Could you check a few things on this model? Use its own coordinates, in mm. Face numbers are marked on the shaded views. A direction names the side the tool comes from. Give positions to 0.01 mm unless a question says otherwise; leave off trailing zeros. Write each loop counter-clockwise with the first axis right and the second up, starting at its lowest first coordinate (ties: lowest second). Pieces come first, ordered by that corner, then holes. Notation, with made-up numbers: (-17, 24) - (22, 24) arc R31 ccw to (22, 62) - close; hole circle Ø4 at (79, 41). An arc over 180 degrees is marked (long way). Write item = value, one per line.
from build123d import *

# Parameters (mm, degrees)
F0_W     = 762
F0_H     = 762
F1_DEPTH = 155.448
F3_DEPTH = 128.016


with BuildPart() as f1:
    # F0 (on Front) → F1 (new body)
    with BuildSketch(Plane.XZ):
        with Locations((-381, 381)):
            Rectangle(F0_W, F0_H)
    extrude(amount=F1_DEPTH)

    # F2 (on face) → F3 (cut)
    with BuildSketch(Plane.XZ.offset(155.448)):
        Polygon((-747.250676, 388.62), (-381, 388.62), (-11.85805, 388.62), (-11.85805, 749.354362), (-747.250676, 749.354362), align=None)
        Polygon((-381, 373.38), (-747.250676, 373.38), (-747.250676, 13.386413), (-11.85805, 13.386413), (-11.85805, 373.38), align=None)
    extrude(amount=-F3_DEPTH, mode=Mode.SUBTRACT)


solid = f1.part
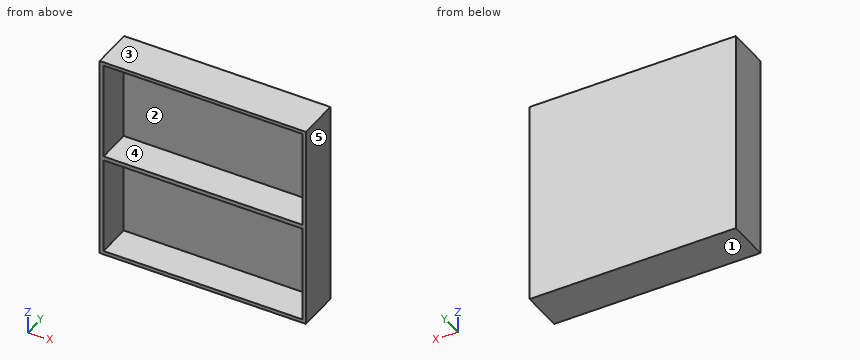
1. Which directions (+Z, -Z, +X, -X, +Y, -Y) give clear straight access to the entire face, cutting with the end or side of a thin tool? Please do the marked faces 1 and 2.
Filled sheet:
face_1 = -Z, +X, -X, +Y, -Y
face_2 = -Y
2. Thinking about a two-plate mould opening in X: for the marked faces 3, 4 and 5, which applies, pulls with the +X half, pulls with the -X half, needs draft (parallel to the pull), parting line crosses it, or undercut?
Filled sheet:
face_3 = needs draft
face_4 = undercut
face_5 = pulls with the +X half
3. For pin 1 (5 mm diameter, centred on x = -117, z = 569.5, fed in from -Y), with a flat end and sliding along its axis, tell me the tip position at first contact or that it passes through.
Filled sheet:
pin_1 = -27.43
4. If we section it at C-C, the plane z = 597.5: Please give me the cut outline in (x, y), and give its area (3 significant figures).
Filled sheet:
outline = (-762, -155.45) - (-747.25, -155.45) - (-747.25, -27.43) - (-11.86, -27.43) - (-11.86, -155.45) - (0, -155.45) - (0, 0) - (-762, 0) - close
area = 24,300 mm2
5. If we section it at B-B, the plane x = -407: Please give me the cut outline in (y, z).
Filled sheet:
outline = (-155.45, 0) - (0, 0) - (0, 762) - (-155.45, 762) - (-155.45, 749.35) - (-27.43, 749.35) - (-27.43, 388.62) - (-155.45, 388.62) - (-155.45, 373.38) - (-27.43, 373.38) - (-27.43, 13.39) - (-155.45, 13.39) - close
6. If we section it at A-A, the plane y = -82.5: Please give me the cut outline in (x, z), and give its area (3 significant figures).
Filled sheet:
outline = (-762, 0) - (0, 0) - (0, 762) - (-762, 762) - close; hole (-747.25, 13.39) - (-11.86, 13.39) - (-11.86, 373.38) - (-747.25, 373.38) - close; hole (-747.25, 388.62) - (-11.86, 388.62) - (-11.86, 749.35) - (-747.25, 749.35) - close
area = 50,600 mm2
7. I need wall thicknesses on line 1 (Z direction, x = -254, y = -79); line 2 (X direction, y = -43.5, z = 633); line 3 (Y direction, x = -551, z = 551). Which ranges of each line are inside material? Lowest first, please.
Filled sheet:
line_1 = 0 to 13.39, 373.38 to 388.62, 749.35 to 762
line_2 = -762 to -747.25, -11.86 to 0
line_3 = -27.43 to 0
